The listing builds one solid part. Answer for the finished solid, in the listing's coordinates (mm). A direction names the side the tool comes from. Coordinates: 2 decimals unless noted, no trailing zeros. Write each loop counter-clockwise with the first axis right and the second up, starting at its lowest first coordinate (ties: lowest second). Pieces come first, ordered by that corner, then holes. Notation, with made-up numbers: M 50,-18.5 L 75,-18.5 A26 cw 75,-3.5 Z; hole C 70.5,6 d4. An arc over 180 degrees is marked long. Answer as CSV lines item,"result". Start each with the question number.
```python
from build123d import *

# Parameters (mm, degrees)
BOSS_EXTRUDE1_DEPTH = 10
SKETCH2_R           = 12.25
BOSS_EXTRUDE2_DEPTH = 23
SKETCH5_R           = 4.7625
BOSS_EXTRUDE3_DEPTH = 10
SKETCH6_R           = 9.337490473
BOSS_EXTRUDE4_DEPTH = 2.54
SKETCH7_R           = 6.793718317
BOSS_EXTRUDE5_DEPTH = 11.43
SKETCH8_R           = 9.337490473
BOSS_EXTRUDE6_DEPTH = 11.43
SKETCH9_R           = 1.5
CUT_EXTRUDE1_DEPTH  = 72.231117539


with BuildPart() as part:
    # Sketch1 → Boss-Extrude1 (new body)
    with BuildSketch(Plane.XY):
        Polygon((14.531817418, -1.969674048), (8.971696472, 11.600086024), (-5.560120947, 13.569760071), (-14.531817418, 1.969674048), (-8.971696472, -11.600086024), (5.560120947, -13.569760071), align=None)
    extrude(amount=BOSS_EXTRUDE1_DEPTH)

    # Sketch2 → Boss-Extrude2 (add)
    with BuildSketch(Plane.XY.offset(10)):
        Circle(SKETCH2_R)
    extrude(amount=BOSS_EXTRUDE2_DEPTH)

    # Sketch5 → Boss-Extrude3 (add)
    with BuildSketch(Plane(origin=(0, 0, 0), x_dir=(-1, 0, 0), z_dir=(0, 0, -1))):
        Circle(SKETCH5_R)
    extrude(amount=BOSS_EXTRUDE3_DEPTH)

    # Sketch6 → Boss-Extrude4 (add)
    with BuildSketch(Plane.XY.offset(33)):
        Circle(SKETCH6_R)
    extrude(amount=BOSS_EXTRUDE4_DEPTH)

    # Sketch7 → Boss-Extrude5 (add)
    with BuildSketch(Plane.XY.offset(35.54)):
        with Locations(Location((0, 0, 0), (0, 0, 180))):
            Circle(SKETCH7_R)
    extrude(amount=BOSS_EXTRUDE5_DEPTH)

    # Sketch8 → Boss-Extrude6 (add)
    with BuildSketch(Plane.XY.offset(46.97)):
        Circle(SKETCH8_R)
    extrude(amount=BOSS_EXTRUDE6_DEPTH)

    # Sketch9 → Cut-Extrude1 (cut, through all)
    with BuildSketch(Plane.XY.offset(58.4)):
        Circle(SKETCH9_R)
    extrude(amount=-CUT_EXTRUDE1_DEPTH, mode=Mode.SUBTRACT)


solid = part.part
```
1) The part is cut by section D-D (x = 10.5). Determine the outline of the cut face in (y, z), then the cut area to 3 significant figures.
2) For a pull along Z with two mould halves and no side action, classify faces 1 (the face through (5, -4.6, 41.2)), 2 (the face through (-1.216, 9.258, 52.605)), 3 (the face through (1, -7, 35.54)), 4 (the face through (0, -6, 0)) as +Z half, -Z half, draft (parallel to the pull), parting line (faces both ways), or undercut.
3) The part is cut by section C-C (x = 0). Determine the outline of the cut face in (y, z), then the cut area to 3 significant figures.
4) Which of the six approach directions +Z, -Z, +X, -X, +Y, -Y give full straight-line access (tool end or side, diameter ignored) to faces 5 (the face through (3.78, -2.9, -4.93)), 6 (the face through (1, -7, 46.97)), 7 (the face through (-1.216, 9.258, 34.252))?
5) Find the intervals of material crossed by line 1 (Y direction, x = 0, z = 23.5); line 2 (Z direction, x = -11.75, y = 1.5); line 3 (Y direction, x = 0, z = 6), in increasing order. Write a range as from..to.
6) Each of these flat-tipped pins is pushed along its axis until it touches: P1, Ø8, axis at y = -4.5, z = 29.5, coming from the -X side; P2, Ø3, axis at x = -11.5, z = 18, coming from the +Y side; P3, Ø1, axis at y = -5.5, z = 0, coming from the +X side. Where does it stop, or does it pass through?
7) The part is cut by section B-B (y = -0.75). Determine the outline of the cut face in (x, z), then the cut area to 3 significant figures.
8) The part is cut by section A-A (z = 7). Determine the outline of the cut face in (x, y), then the cut area to 3 significant figures.
Completed:
1,outline,"M -7.18,0 L 7.87,0 L 7.87,10 L 6.31,10 L 6.31,33 L -6.31,33 L -6.31,10 L -7.18,10 Z"
1,area,"441 mm²"
2,face 1,"undercut"
2,face 2,"draft"
2,face 3,"undercut"
2,face 4,"-Z half"
3,outline,"M -12.82,0 L -4.76,0 L -4.76,-10 L -1.5,-10 L -1.5,58.4 L -9.34,58.4 L -9.34,46.97 L -6.79,46.97 L -6.79,35.54 L -9.34,35.54 L -9.34,33 L -12.25,33 L -12.25,10 L -12.82,10 Z; M 1.5,-10 L 4.76,-10 L 4.76,0 L 12.82,0 L 12.82,10 L 12.25,10 L 12.25,33 L 9.34,33 L 9.34,35.54 L 6.79,35.54 L 6.79,46.97 L 9.34,46.97 L 9.34,58.4 L 1.5,58.4 Z"
3,area,"1,130 mm²"
4,face 5,"-Z"
4,face 6,"none"
4,face 7,"+Z"
5,line 1,"-12.25..-1.5, 1.5..12.25"
5,line 2,"0..33"
5,line 3,"-12.82..-1.5, 1.5..12.82"
6,P1,"x = -12.24"
6,P2,"y = 7.08"
6,P3,"x = 12.19"
7,outline,"M -13.42,0 L -4.7,0 L -4.7,-10 L -1.3,-10 L -1.3,58.4 L -9.31,58.4 L -9.31,46.97 L -6.75,46.97 L -6.75,35.54 L -9.31,35.54 L -9.31,33 L -12.23,33 L -12.23,10 L -13.42,10 Z; M 1.3,-10 L 4.7,-10 L 4.7,0 L 14.03,0 L 14.03,10 L 12.23,10 L 12.23,33 L 9.31,33 L 9.31,35.54 L 6.75,35.54 L 6.75,46.97 L 9.31,46.97 L 9.31,58.4 L 1.3,58.4 Z"
7,area,"1,170 mm²"
8,outline,"M -14.53,1.97 L -8.97,-11.6 L 5.56,-13.57 L 14.53,-1.97 L 8.97,11.6 L -5.56,13.57 Z; hole C 0,0 d3"
8,area,"552 mm²"
